from build123d import *

# Parameters (mm, degrees)
F0_R      = 19.05
F1_DEPTH  = 2.54
F2_R      = 6.35
F3_DEPTH  = 25.4
F5_DEPTH  = 7.62
F7_DEPTH  = 7.62
F9_DEPTH  = 25.4
F11_DEPTH = 25.4
F13_DEPTH = 25.4
F15_DEPTH = 25.4
F16_W     = 19.05
F16_H     = 6.35
F17_DEPTH = 50.8
F18_W     = 19.05
F18_H     = 6.35
F19_DEPTH = 50.8
F21_DEPTH = 50.8
F23_DEPTH = 5.08
F25_DEPTH = 25.4
F26_R     = 9.525
F27_DEPTH = 76.2
F29_W     = 10
F29_H     = 10
F30_DEPTH = 71.12
F28_W     = 10
F28_H     = 10
F31_DEPTH = 71.12
F33_R     = 3.3655
F32_R     = 3.3655
F34_DEPTH = 25.4


with BuildPart() as f1:
    # F0 (on Top) → F1 (new body)
    with BuildSketch(Plane.XY):
        Circle(F0_R)
    extrude(amount=F1_DEPTH)

    # F2 (on face) → F3 (join)
    with BuildSketch(Plane.XY.offset(2.54)):
        Circle(F2_R)
    extrude(amount=F3_DEPTH)

    # F4 (on Right) → F5 (join)
    with BuildSketch(Plane.YZ):
        Polygon((-6.3969814219, 31.7939482629), (-6.3969814219, 27.4019930512), (12.6530185781, 27.4019930512), (12.6530185781, 35.0219930512), align=None)
    extrude(amount=F5_DEPTH)

    # F6 (on face) → F7 (join)
    with BuildSketch(Plane(origin=(0, 0, 0), x_dir=(0, -1, 0), z_dir=(-1, 0, 0))):
        Polygon((-12.6530185781, 35.0219930512), (-12.6530185781, 27.4019930512), (6.3969814219, 27.4019930512), (6.3969814219, 31.7939482629), align=None)
    extrude(amount=F7_DEPTH)

    # F8 (on Right) → F9 (join)
    with BuildSketch(Plane.YZ):
        Polygon((-15.9447137266, 30.0753582269), (15.3388162634, 35.4978347242), (35.2311320603, 39.2411798239), (31.9399436585, 51.2647326185), (-18.1137043255, 42.5887702229), align=None)
    extrude(amount=F9_DEPTH)

    # F10 (on face) → F11 (join)
    with BuildSketch(Plane(origin=(0, 0, 0), x_dir=(0, -1, 0), z_dir=(-1, 0, 0))):
        Polygon((-31.9399436585, 51.2647326185), (-35.2311320603, 39.2411798239), (15.9447137266, 30.0753582269), (18.1137043255, 42.5887702229), align=None)
    extrude(amount=F11_DEPTH)

    # F12 (on Right) → F13 (join)
    with BuildSketch(Plane.YZ):
        Polygon((-19.1909428686, 46.8793660402), (-17.8339676882, 40.6760509298), (-13.3405660695, 40.6760509298), (-14.9027385279, 47.8174107397), align=None)
    extrude(amount=F13_DEPTH)

    # F14 (on face) → F15 (join)
    with BuildSketch(Plane(origin=(0, 0, 0), x_dir=(0, -1, 0), z_dir=(-1, 0, 0))):
        Polygon((13.3405660695, 40.6760509298), (17.8339676882, 40.6760509298), (19.1909428686, 46.8793660402), (14.9027385279, 47.8174107397), align=None)
    extrude(amount=F15_DEPTH)

    # F16 (on face) → F17 (cut)
    with BuildSketch(Plane(origin=(0, -8.528003266, -1.8655007144), x_dir=(1, 0, 0), z_dir=(0, -0.9769000174, -0.2136968788))):
        with Locations((-15.875, 46.7224980926)):
            Rectangle(F16_W, F16_H)
    extrude(amount=-F17_DEPTH, mode=Mode.SUBTRACT)

    # F18 (on face) → F19 (cut)
    with BuildSketch(Plane(origin=(0, -8.528003266, -1.8655007144), x_dir=(1, 0, 0), z_dir=(0, -0.9769000174, -0.2136968788))):
        with Locations((15.875, 46.7224980926)):
            Rectangle(F18_W, F18_H)
    extrude(amount=-F19_DEPTH, mode=Mode.SUBTRACT)

    # F20 (on face) → F21 (cut)
    with BuildSketch(Plane(origin=(0, -8.528003266, -1.8655007144), x_dir=(1, 0, 0), z_dir=(0, -0.9769000174, -0.2136968788))):
        Polygon((3.175, 49.8974980926), (0, 49.8974980926), (-3.175, 49.8974980926), (-3.175, 43.5474980926), (3.175, 43.5474980926), align=None)
    extrude(amount=-F21_DEPTH, mode=Mode.SUBTRACT)

    # F22 (on face) → F23 (join)
    with BuildSketch(Plane(origin=(0, -7.6950725058, 44.3946657275), x_dir=(1, 0, 0), z_dir=(0, -0.1707866613, 0.9853080312))):
        Polygon((3.175, 40.2260155302), (0, 40.2260155302), (-3.175, 40.2260155302), (-3.175, 36.4160155302), (3.175, 36.4160155302), align=None)
    extrude(amount=F23_DEPTH)

    # F24 (on face) → F25 (cut)
    with BuildSketch(Plane(origin=(0, 39.6350161643, 6.870066891), x_dir=(-1, 0, 0), z_dir=(0, 0.9853080312, 0.1707866613))):
        Polygon((1.27, 50.1366364249), (0, 50.1366364249), (-1.27, 50.1366364249), (-1.27, 48.8666364249), (1.27, 48.8666364249), align=None)
    extrude(amount=-F25_DEPTH, mode=Mode.SUBTRACT)

    # F26 (on face) → F27 (join)
    with BuildSketch(Plane(origin=(0, -10.4186318197, -1.8058955046), x_dir=(1, 0, 0), z_dir=(0, -0.9853080312, -0.1707866613))):
        with Locations((-16.5175776929, 50.3802224994)):
            Circle(F26_R)
        with Locations((16.3266230375, 50.3802224994)):
            Circle(F26_R)
    extrude(amount=-F27_DEPTH)

    # F29 (on face) → F30 (cut)
    with BuildSketch(Plane(origin=(0, 64.6618401563, 11.2080480889), x_dir=(-1, 0, 0), z_dir=(0, 0.9853080312, 0.1707866613))):
        with Locations((16.5175776929, 50.3802224994)):
            Rectangle(F29_W, F29_H)
    extrude(amount=-F30_DEPTH, mode=Mode.SUBTRACT)

    # F28 (on face) → F31 (cut)
    with BuildSketch(Plane(origin=(0, 64.6618401563, 11.2080480889), x_dir=(-1, 0, 0), z_dir=(0, 0.9853080312, 0.1707866613))):
        with Locations((-16.3266230375, 50.3802224994)):
            Rectangle(F28_W, F28_H)
    extrude(amount=-F31_DEPTH, mode=Mode.SUBTRACT)

    # F33 (on face) + F32 (on face) → F34 (cut)
    with BuildSketch(Plane(origin=(0, -10.4186318197, -1.8058955046), x_dir=(1, 0, 0), z_dir=(0, -0.9853080312, -0.1707866613))):
        with Locations((16.3266230375, 50.3802224994)):
            Circle(F33_R)
    with BuildSketch(Plane(origin=(0, -10.4186318197, -1.8058955046), x_dir=(1, 0, 0), z_dir=(0, -0.9853080312, -0.1707866613))):
        with Locations((-16.5175776929, 50.3802224994)):
            Circle(F32_R)
    extrude(amount=-F34_DEPTH, mode=Mode.SUBTRACT)


solid = f1.part
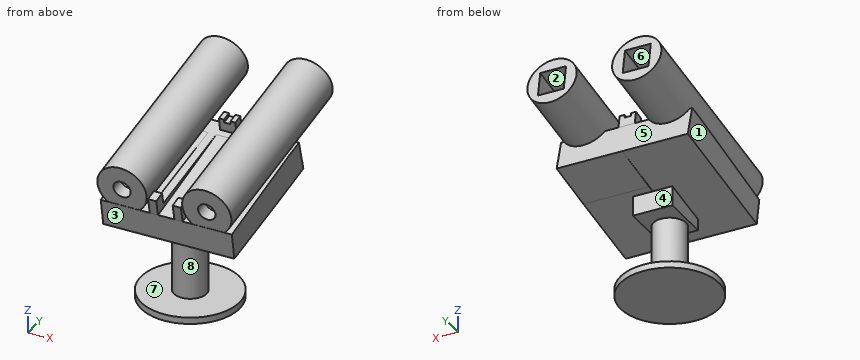
Design review of the part built by this model. Coordinates are the model's own, in mm. Face numbers are marked on the shaded views. A direction names the side the tool comes from. Give positions to 0.01 mm unless a question says otherwise; leave off trailing zeros. Loops run counter-clockwise (first coordinate to the right, second up) from the corner with the lowest first, then second, coordinate; pieces in that order, holes last. Notation, with made-up numbers: (62.5, 83.5) -> (105.5, 83.5) arc R25 cw to (105.5, 116.5) -> close; hole circle Ø10 at (-25.5, -32). An arc over 180 degrees is marked (long way). One line per question, with ' | ' between items. Start each with the question number.
(1) For line 1 (X direction, y = 50, z = 64.5); line 2 (Z direction, x = -14, y = 2.5); line 3 (Z direction, x = -12, y = 4), list the stretches that pass through material, from the lowest coordinate up.
(2) We need section A-A (x = -5). State the section outline as (y, z) points, and give its area (3 significant figures).
(3) We need section B-B (y = -2). State how many separate pieces and enclosed holes the cut face has, and give its area (3 significant figures).
(4) Draft analysis for pull direction X (two halves, no side actions). For the marked faces 6, 7 and 8, state which applies: +X half, -X half, draft (parallel to the pull), parting line (faces both ways), or undercut.
(5) For the marked faces 1, 2, 3, 4 and 5, list the 3-axis set-ups (+Z, -Z, +X, -X, +Y, -Y) from which the entire face can be reached by the end or side of a thin tool; tool diameter is ignored.
(6) Insertion check: P1, Ø3, axis at x = -17, z = 52.5, coming from the -Y side; P2, Ø4, axis at x = 9.5, y = -6.5, coming from the +Z side; P3, Ø7.5, axis at y = -2, z = 44, coming from the -X side. Each pin has a flat end and moves straight along its axis. Give the tip position at first contact, or say it passes through.
The answers:
1) line 1: x = -24.84 to -21.52, -11.52 to -8.2, 8 to 11.33, 21.33 to 24.65 | line 2: z = 0 to 2.54, 33.38 to 46.49, 56.64 to 60.89 | line 3: z = 0 to 2.54, 33.65 to 46.75, 56.9 to 60.34
2) outline: (-19.19, 46.88) -> (-17.83, 40.68) -> (-17.78, 40.68) -> (-15.94, 30.08) -> (-6.4, 31.79) -> (-6.4, 27.4) -> (-3.91, 27.4) -> (-3.91, 2.54) -> (-18.38, 2.54) -> (-18.38, 0) -> (18.38, 0) -> (18.38, 2.54) -> (3.91, 2.54) -> (3.91, 27.4) -> (12.65, 27.4) -> (12.65, 35.02) -> (-5.51, 31.94) -> (35.23, 39.24) -> (31.94, 51.26) -> (-13.92, 43.32) -> (-14.9, 47.82) -> close | area: 1,070 mm^2
3) separate pieces: 1 | enclosed holes: 2 | area: 1,390 mm^2
4) face 6: undercut | face 7: draft | face 8: parting line
5) face 1: -Z, -X, +Y | face 2: none | face 3: +X, -X, -Y | face 4: +X, -X, +Y | face 5: +Y
6) P1: stops at y = -20.09 | P2: stops at z = 58.39 | P3: stops at x = -25.58
